from build123d import *

# Parameters (mm, degrees)
SKETCH_1_W      = 60
SKETCH_1_H      = 4
SKETCH_3_R      = 5
EXTRUDE_2_DEPTH = 30
SKETCH_5_W      = 110
SKETCH_5_H      = 130
EXTRUDE_3_DEPTH = 10


with BuildPart() as part:
    # 草图1 → 旋转3 (revolve)
    with BuildSketch(Plane(origin=(0, 0, 0), x_dir=(1, 0, 0), z_dir=(0, 1, 0)), mode=Mode.PRIVATE) as revolve_3_sk:
        with Locations((0, 2)):
            Rectangle(SKETCH_1_W, SKETCH_1_H)
    revolve(revolve_3_sk.sketch.rotate(Axis((-30, 0, 0), (1, 0, 0)), 180), axis=Axis((-30, 0, 0), (1, 0, 0)))

    # 草图3 → 凸台-拉伸2 (add)
    with BuildSketch(Plane(origin=(0, 0, 0), x_dir=(1, 0, 0), z_dir=(0, 1, 0))):
        with Locations(Location((0, 0, 0), (0, 0, 270))):
            Circle(SKETCH_3_R)
    extrude(amount=-EXTRUDE_2_DEPTH)

    # 草图5 → 凸台-拉伸3 (add)
    with BuildSketch(Plane.XZ.offset(30)):
        Rectangle(SKETCH_5_W, SKETCH_5_H)
    extrude(amount=EXTRUDE_3_DEPTH)


solid = part.part
Source: CAD feature listing. Evaluate the final solid. Frame: model axes, mm. A direction names the side the tool comes from. Coordinates: 2 decimals unless noted, no trailing zeros. Loops run counter-clockwise (first coordinate to the right, second up) from the corner with the lowest first, then second, coordinate; pieces in that order, holes last. Notation, with made-up numbers: (-29.75, 86.5) -> (9.25, 86.5) arc R16 ccw to (9.25, 90.5) -> close; hole circle Ø8 at (69, -1.75). An arc over 180 degrees is marked (long way). Answer in a Markdown table with one row per item. Add a question column.
Q1. Section B-B on z = 0. Return the cut outline in (x, y).
Q2. Section A-A on x = 21.5. Return the cut outline in (y, z), and give its area (3 significant figures).
Q3. Section D-D on y = -7. Return the cut outline in (x, z), and give its area (3 significant figures).
Q4. Ray query, line 1 along Y through (x, z) = (49, -44.5); line 2 along Z through (x, y) = (-22.5, 2); line 3 along Z through (x, y) = (-21, 2.5). Return the intervals inside material, ascending.
Q5. Section C-C on x = 0. Return the cut outline in (y, z), and give its area (3 significant figures).
Q6. Pull-direction query (Y, two-part tool) for faces 1 (the face through (30, 0, 0)), 2 (the face through (0.42, 3.905, -0.867)), 3 (the face through (-1, -40, 1)); classes: pulls with the +Y half, pulls with the -Y half, needs draft (parallel to the pull), parting line crosses it, or undercut.
Q7. Contact query for flat-ended pins moving along their axis: pin 1 Ø4 at (y, z) = (1, 0.5) entering from -X; pin 2 Ø0.5 at (x, z) = (-0.5, 4.5) entering from +Y; pin 3 Ø8 at (x, y) = (-3.5, -8) entering from +Z. Output: stop coordinate, or through.
Q8. Reachability of faces 4 (the face through (-1, -35, 65)), 5 (the face through (-30, 0, 0)), 6 (the face through (-4.88, -14.79, -1.08)) from +Z, -Z, +X, -X, +Y, -Y: full face, straight path, thin tool, end or side. Return the list, or none.
Computed values:
| question | item | result |
|---|---|---|
| 1 | outline | (-55, -40) -> (55, -40) -> (55, -30) -> (5, -30) -> (5, -4) -> (30, -4) -> (30, 4) -> (-30, 4) -> (-30, -4) -> (-5, -4) -> (-5, -30) -> (-55, -30) -> close |
| 2 | outline | (-40, -65) -> (-30, -65) -> (-30, 65) -> (-40, 65) -> close; circle Ø8 at (0, 0) |
| 2 | area | 1,350 mm^2 |
| 3 | outline | circle Ø10 at (0, 0) |
| 3 | area | 78.5 mm^2 |
| 4 | line 1 | y = -40 to -30 |
| 4 | line 2 | z = -3.46 to 3.46 |
| 4 | line 3 | z = -3.12 to 3.12 |
| 5 | outline | (-40, -65) -> (-30, -65) -> (-30, -5) -> (0, -5) -> (0, -4) arc R4 ccw to (0, 4) -> (0, 5) -> (-30, 5) -> (-30, 65) -> (-40, 65) -> close |
| 5 | area | 1,630 mm^2 |
| 6 | face 1 | needs draft |
| 6 | face 2 | undercut |
| 6 | face 3 | pulls with the -Y half |
| 7 | pin 1 | stops at x = -30 |
| 7 | pin 2 | stops at y = 0 |
| 7 | pin 3 | stops at z = 5 |
| 8 | face 4 | +Z, +X, -X, +Y, -Y |
| 8 | face 5 | +Z, -Z, -X, +Y |
| 8 | face 6 | none |
